```python
from build123d import *

# Parameters (mm, degrees)
F0_W      = 139.7
F0_H      = 38.1
F1_DEPTH  = 1828.8
F3_W      = 331.3202857971
F3_H      = 260.5838701129
F4_DEPTH  = 101.6
F7_W      = 1553.4552037716
F7_H      = 1155.3529500961
F8_DEPTH  = 762
F9_R      = 6.35
F10_DEPTH = 38.101


with BuildPart() as f1:
    # F0 (on Front) → F1 (new body)
    with BuildSketch(Plane.XZ):
        with Locations((69.85, 19.05)):
            Rectangle(F0_W, F0_H)
    extrude(amount=F1_DEPTH)

    # F3 (on face) → F4 (cut)
    with BuildSketch(Plane(origin=(984.25, -984.25, 0), x_dir=(-0.7071067812, -0.7071067812, 0), z_dir=(-0.7071067812, 0.7071067812, 0))):
        with Locations((1222.6701974869, 7.0506222546)):
            Rectangle(F3_W, F3_H)
    extrude(amount=F4_DEPTH, mode=Mode.SUBTRACT)

    # F7 (on face) → F8 (cut)
    with BuildSketch(Plane(origin=(-216.4381016486, -216.4381016486, 0), x_dir=(0.7071067812, -0.7071067812, 0), z_dir=(-0.7071067812, -0.7071067812, 0))):
        with Locations((614.4417077303, -181.5140247345)):
            Rectangle(F7_W, F7_H)
    extrude(amount=-F8_DEPTH, mode=Mode.SUBTRACT)

    # F9 (on face) → F10 (cut, through all)
    with BuildSketch(Plane.XY.offset(38.1)):
        with Locations((69.85, -566.2262032972)):
            Circle(F9_R)
    extrude(amount=-F10_DEPTH, mode=Mode.SUBTRACT)


solid = f1.part
```
Work out the finished part from the listing and answer in its coordinate system (mm). Round coordinates to 2 decimals unless told otherwise and drop trailing zeros. Write each loop counter-clockwise with the first axis right and the second up, starting at its lowest first coordinate (ties: lowest second). Pieces come first, ordered by that corner, then holes.
1) A cutting plane is placed at B-B on x = 19. Determine the outline of the cut face in (y, z), and give its area (3 significant figures).
2) A cutting plane is placed at A-A on z = 25. Determine the outline of the cut face in (x, y).
3) A cutting plane is placed at C-C on x = 111.5. Determine the outline of the cut face in (y, z).
4) Consider probe 1 along Y at (x, z) = (69, 11); probe 2 along Y at (x, z) = (70, 17.5); probe 3 along Y at (x, z) = (78, 22). Determine where each line is inside the solid, lowest interval first.
Entries:
1. outline: (-1805.82, 0) - (-451.88, 0) - (-451.88, 38.1) - (-1805.82, 38.1) - close
1. area: 51,600 mm2
2. outline: (0, -1824.82) - (139.7, -1685.12) - (139.7, -572.58) - (0, -432.88) - close; hole circle Ø12.7 at (69.85, -566.23)
3. outline: (-1713.32, 0) - (-544.38, 0) - (-544.38, 38.1) - (-1713.32, 38.1) - close
4. probe 1: y = -1755.82 to -572.52, -559.93 to -501.88
4. probe 2: y = -1754.82 to -572.57, -559.88 to -502.88
4. probe 3: y = -1746.82 to -510.88
